Read the model definition and answer for the solid it produces. Units are mm, in the model's axes. A direction names the side the tool comes from. Coordinates: 2 decimals unless noted, no trailing zeros. Loops run counter-clockwise (first coordinate to the right, second up) from the corner with the lowest first, then second, coordinate; pieces in that order, holes last. Notation, with made-up numbers: M 27.25,80 L 34.25,80 A23 ccw 34.25,99 Z; hole C -27,87 d5. An arc over 180 degrees is marked long. Use one line per item in the form item = value. Start each with the question number.
1. The part is cut by section C-C (x = 47). Give the vertices of the cut face in (y, z), plus the area to 3 significant figures.
2. The part is cut by section D-D (x = 14). Give the vertices of the cut face in (y, z), plus the area to 3 significant figures.
3. The part is cut by section B-B (z = 5.25). Give the vertices of the cut face in (x, y).
4. A tool of negligible diameter and unlimited length cuts with its end or side. For faces 1 (the conical face through (-48.85, 0.01, 2.19)), 2 (the flat face through (-24.6, -51, 5)), 3 (the flat face through (50, -88, 5)), from which of +Z, -Z, +X, -X, +Y, -Y can it reach the whole face along a straight path? Write none if from no direction.
5. For a pull along X with two mould halves and no side action, classify faces 4 (the flat face through (-50, -60, 5)), 5 (the conical face through (39.673, -84.745, 2.188)), 6 (the flat face through (12, -21.685, 5)) as released by +X, released by -X, zero draft, split by the parting line, or undercut.
6. Find the intervals of material crossed by probe 1 along X at (y, z) = (-3.5, 8.5); probe 2 along Y at (x, z) = (40, 7.25); probe 3 along X at (y, z) = (-46, 9), in increasing order. Write a range as [from, to].
7. The part is cut by section A-A (x = 0). Give the vertices of the cut face in (y, z).
8. Flat-ended cylindrical pins translate along their axes: pin 1 (1 mm diameter, centred on x = -39, z = 2, fed in from +Y); pin 2 (6 mm diameter, centred on x = 40, y = -87.24, fed in from -Z); pin 3 (5 mm diameter, centred on y = -72, z = 6, fed in from -X). Find the tip coordinate at first contact, or state that the pin passes through.
from build123d import *

# Parameters (mm, degrees)
BOSS_EXTRUDE1_DEPTH                             = 10
CSK_FOR_M4_FLAT_HEAD_MACHINE_SCREW1_D           = 4.8
CSK_FOR_M4_FLAT_HEAD_MACHINE_SCREW1_CSINK_D     = 9.4
CSK_FOR_M4_FLAT_HEAD_MACHINE_SCREW1_CSINK_ANGLE = 90
SKETCH6_W                                       = 74.6
SKETCH6_H                                       = 57.3
CUT_EXTRUDE1_DEPTH                              = 15


with BuildPart() as part:
    # Sketch1 → Boss-Extrude1 (new body)
    with BuildSketch(Plane(origin=(0, 0, 0), x_dir=(-1, 0, 0), z_dir=(0, 0, 1))):
        with BuildLine():
            Line((-50, 21.685248442), (-50, 97.235188276))
            Line((-50, 97.235188276), (50, 97.235188276))
            Line((50, 97.235188276), (50, 21.685248442))
            ThreePointArc((50, 21.685248442), (0, -54.5), (-50, 21.685248442))
        make_face()
    extrude(amount=BOSS_EXTRUDE1_DEPTH)

    # CSK for M4 Flat Head Machine Screw1 (through all)
    with Locations(Plane(origin=(47, -1.685248442, 0), x_dir=(-1, 0, 0), z_dir=(0, 0, -1))):
        with Locations((0, 0), (94, 0), (87, -85.549939834), (7, -85.549939834)):
            CounterSinkHole(CSK_FOR_M4_FLAT_HEAD_MACHINE_SCREW1_D / 2, CSK_FOR_M4_FLAT_HEAD_MACHINE_SCREW1_CSINK_D / 2, counter_sink_angle=CSK_FOR_M4_FLAT_HEAD_MACHINE_SCREW1_CSINK_ANGLE)

    # Sketch6 → Cut-Extrude1 (cut)
    with BuildSketch(Plane.XY.offset(10)):
        with Locations((12.7, -50.335248442)):
            Rectangle(SKETCH6_W, SKETCH6_H)
    extrude(amount=-CUT_EXTRUDE1_DEPTH, mode=Mode.SUBTRACT)


solid = part.part
Computed values:
q1.outline = M -97.24,0 L -78.99,0 L -78.99,10 L -97.24,10 Z; M -21.69,0 L -6.39,0 L -4.09,2.3 L -4.09,10 L -21.69,10 Z; M 0.71,2.3 L 3.01,0 L 27.59,0 L 27.59,10 L 0.71,10 Z
q1.area = 622 mm²
q2.outline = M -97.24,0 L -78.99,0 L -78.99,10 L -97.24,10 Z; M -21.69,0 L 52.67,0 L 52.67,10 L -21.69,10 Z
q2.area = 926 mm²
q3.outline = M -50,-97.24 L 50,-97.24 L 50,-78.99 L -24.6,-78.99 L -24.6,-21.69 L 50,-21.69 A54.5 ccw long -50,-21.69 Z; hole C -47,-1.69 d4.8; hole C -40,-87.24 d4.8; hole C 40,-87.24 d4.8; hole C 47,-1.69 d4.8
q4.face_1 = -Z
q4.face_2 = +Z, -Z, +X
q4.face_3 = +Z, -Z, +X, -Y
q5.face_4 = released by -X
q5.face_5 = undercut
q5.face_6 = zero draft
q6.probe_1 = [-54.39, -48.57], [-45.43, 45.43], [48.57, 54.39]
q6.probe_2 = [-97.24, -89.64], [-84.84, -78.99], [-21.69, 37.02]
q6.probe_3 = [-50, -24.6]
q7.outline = M -97.24,0 L -78.99,0 L -78.99,10 L -97.24,10 Z; M -21.69,0 L 54.5,0 L 54.5,10 L -21.69,10 Z
q8.pin_1 = 38.57
q8.pin_2 = 1.7
q8.pin_3 = -50
